For this review, take the finished solid that the model builds, in its own axes (mm). Coordinates: 2 decimals unless noted, no trailing zeros. Write each loop counter-clockwise with the first axis right and the second up, starting at its lowest first coordinate (ties: lowest second). Pieces come first, ordered by that corner, then holes. Notation, with made-up numbers: (71.25, 42.5) - (124.25, 42.5) arc R19 ccw to (124.25, 52.5) - close; hole circle Ø11 at (87, 8.5). An arc over 180 degrees is marked (long way). Use one line per item in the form item = value. Start each with the question number.
1) We need section C-C (y = 1.1). Count the separate pieces of the cut face and the enclosed holes in it, plus the area to 3 significant figures.
2) Insertion check: P1, Ø4, axis at x = 34.19, z = 9.19, coming from the -Y side; P2, Ø2.5, axis at x = -22, z = -12, coming from the -Y side. Each pin has a flat end and moves straight along its axis. Give the tip position at first contact, or say it passes through.
3) We need section B-B (x = -11). Give the boundary of the cut face in (y, z).
4) For L1, parallel to Z at x = -22, y = 2.05 (3 decimals); L2, parallel to Z at x = 16, y = 1.1; L3, parallel to Z at x = 12, y = 2.1 (3 decimals), list the stretches that pass through material, from the lowest coordinate up. Write a range as from..to.
5) We need section A-A (x = 12). Give the boundary of the cut face in (y, z) (3 decimals), plus the area to 4 significant figures.
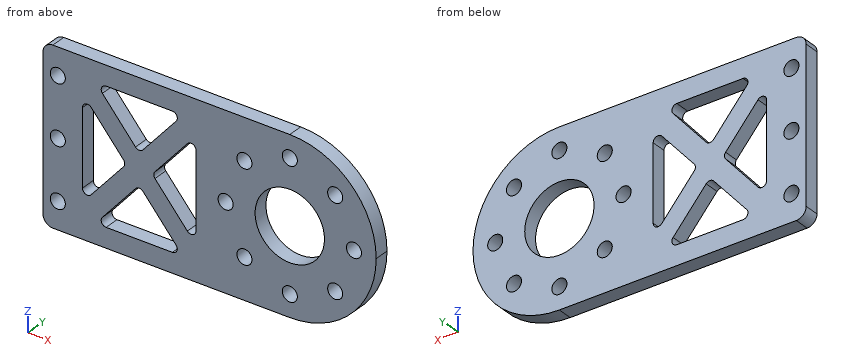
```python
from build123d import *

# Parameters (mm, degrees)
EXTRUDE_1_DEPTH     = 3
SKETCH_2_R          = 7.025
CUT_EXTRUDE_1_DEPTH = 4
SKETCH_4_R          = 1.525
CUT_EXTRUDE_3_DEPTH = 4
FILLET_2_R          = 2
CUT_EXTRUDE_6_DEPTH = 4
SKETCH_10_R         = 1.525
CUT_EXTRUDE_8_DEPTH = 4
FILLET_7_R          = 1


with BuildPart() as part:
    # 草图1 → 凸台-拉伸1 (new body)
    with BuildSketch(Plane(origin=(0, 0, 0), x_dir=(1, 0, 0), z_dir=(0, 1, 0))):
        with BuildLine():
            Line((-25, 17.5), (-25, -17.5))
            Line((-25, -17.5), (25, -17.5))
            ThreePointArc((25, -17.5), (7.5, 0), (25, 17.5))
            Line((25, 17.5), (-25, 17.5))
        make_face()
        with BuildLine():
            ThreePointArc((25, 17.5), (7.5, 0), (25, -17.5))
            Line((25, -17.5), (25, 17.5))
        make_face()
        with BuildLine():
            Line((25, 17.5), (25, -17.5))
            ThreePointArc((25, -17.5), (37.374368671, -12.374368671), (42.5, 0))
            ThreePointArc((42.5, 0), (37.374368671, 12.374368671), (25, 17.5))
        make_face()
    extrude(amount=EXTRUDE_1_DEPTH)

    # 草图2 → 切除-拉伸1 (cut, through all)
    with BuildSketch(Plane(origin=(0, 3, 0), x_dir=(1, 0, 0), z_dir=(0, 1, 0))):
        with Locations((25, 0)):
            Circle(SKETCH_2_R)
    extrude(amount=-CUT_EXTRUDE_1_DEPTH, mode=Mode.SUBTRACT)

    # 草图4 → 切除-拉伸3 (cut, through all)
    with BuildSketch(Plane(origin=(0, 3, 0), x_dir=(1, 0, 0), z_dir=(0, 1, 0))):
        with Locations((25, 13)):
            Circle(SKETCH_4_R)
        with Locations((34.192388155, 9.192388155)):
            Circle(SKETCH_4_R)
        with Locations((38, 0)):
            Circle(SKETCH_4_R)
        with Locations((34.192388155, -9.192388155)):
            Circle(SKETCH_4_R)
        with Locations((25, -13)):
            Circle(SKETCH_4_R)
        with Locations((15.807611845, -9.192388155)):
            Circle(SKETCH_4_R)
        with Locations((12, 0)):
            Circle(SKETCH_4_R)
        with Locations((15.807611845, 9.192388155)):
            Circle(SKETCH_4_R)
    extrude(amount=-CUT_EXTRUDE_3_DEPTH, mode=Mode.SUBTRACT)

    # 圆角2
    fillet_2_edges = [part.edges().sort_by_distance(p)[0] for p in [
        (-25, 1.5, 17.5),
        (-25, 1.5, -17.5),
    ]]
    fillet(fillet_2_edges, radius=FILLET_2_R)

    # 草图7 → 切除-拉伸6 (cut, through all)
    with BuildSketch(Plane(origin=(0, 3, 0), x_dir=(1, 0, 0), z_dir=(0, 1, 0))):
        Polygon((3.372718837, 13.5), (-14.372718837, 13.5), (-5.5, 3.084199626), align=None)
        Polygon((-2.872718837, 0), (6, -10.415800374), (6, 10.415800374), align=None)
        Polygon((-5.5, -3.084199626), (-14.372718837, -13.5), (3.372718837, -13.5), align=None)
        Polygon((-17, 10.415800374), (-17, -10.415800374), (-8.127281163, 0), align=None)
    extrude(amount=-CUT_EXTRUDE_6_DEPTH, mode=Mode.SUBTRACT)

    # 草图10 → 切除-拉伸8 (cut, through all)
    with BuildSketch(Plane(origin=(0, 3, 0), x_dir=(1, 0, 0), z_dir=(0, 1, 0))):
        with Locations((-22, 0)):
            Circle(SKETCH_10_R)
        with Locations((-22, 12)):
            Circle(SKETCH_10_R)
        with Locations((-22, -12)):
            Circle(SKETCH_10_R)
    extrude(amount=-CUT_EXTRUDE_8_DEPTH, mode=Mode.SUBTRACT)

    # 圆角7
    fillet_7_edges = [part.edges().sort_by_distance(p)[0] for p in [
        (-17, 1.5, 10.415800374),
        (-17, 1.5, -10.415800374),
        (-8.127281163, 1.5, 0),
        (-5.5, 1.5, -3.084199626),
        (-14.372718837, 1.5, -13.5),
        (3.372718837, 1.5, -13.5),
        (-14.372718837, 1.5, 13.5),
        (-5.5, 1.5, 3.084199626),
        (3.372718837, 1.5, 13.5),
        (-2.872718837, 1.5, 0),
        (6, 1.5, -10.415800374),
        (6, 1.5, 10.415800374),
    ]]
    fillet(fillet_7_edges, radius=FILLET_7_R)


solid = part.part
```
Determined:
q1.separate_pieces = 1
q1.enclosed_holes = 16
q1.area = 1,640 mm²
q2.P1 = 0
q2.P2 = through
q3.outline = (0, -17.5) - (3, -17.5) - (3, -13.5) - (0, -13.5) - close; (0, -9.54) - (3, -9.54) - (3, -3.37) - (0, -3.37) - close; (0, 3.37) - (3, 3.37) - (3, 9.54) - (0, 9.54) - close; (0, 13.5) - (3, 13.5) - (3, 17.5) - (0, 17.5) - close
q4.L1 = -17.5..-13.525, -10.475..-1.525, 1.525..10.475, 13.525..17.5
q4.L2 = -17.5..-10.71, -7.68..7.68, 10.71..17.5
q4.L3 = -17.5..-1.525, 1.525..17.5
q5.outline = (0, -17.5) - (3, -17.5) - (3, -1.525) - (0, -1.525) - close; (0, 1.525) - (3, 1.525) - (3, 17.5) - (0, 17.5) - close
q5.area = 95.85 mm²
